```python
from build123d import *

# Parameters (mm, degrees)
BOSS_EXTRUDE1_DEPTH             = 2
BOSS_EXTRUDE3_DEPTH             = 8
BOSS_EXTRUDE2_REACH             = 28
BOSS_EXTRUDE2_DIRECTION_2_REACH = 28
TAP_DRILL_FOR_M3X0_5_TAP1_D     = 2.5
TAP_DRILL_FOR_M3X0_5_TAP1_DEPTH = 8


with BuildPart() as part:
    # Sketch1 → Boss-Extrude1 (new body)
    with BuildSketch(Plane(origin=(0, 0, 0), x_dir=(1, 0, 0), z_dir=(0, 1, 0))):
        with BuildLine():
            Line((-26, 0), (-26, -19))
            Line((-26, -19), (26, -19))
            Line((26, -19), (26, 0))
            ThreePointArc((26, 0), (0, 26), (-26, 0))
        make_face()
    extrude(amount=BOSS_EXTRUDE1_DEPTH)

    # Sketch1<3> → Boss-Extrude3 (add)
    with BuildSketch(Plane(origin=(0, 0, 0), x_dir=(1, 0, 0), z_dir=(0, 1, 0))):
        with BuildLine():
            ThreePointArc((26, 0), (0, 26), (-26, 0))
            Line((-26, 0), (-26, -19))
            Line((-26, -19), (26, -19))
            Line((26, -19), (26, 0))
        make_face()
    extrude(amount=BOSS_EXTRUDE3_DEPTH)

    # Boss-Extrude2: up to this face of the body (flat: up to its plane)
    boss_extrude2_end = Plane(part.part.faces().sort_by_distance((26, 4, 9.5))[0])
    # Sketch3 → Boss-Extrude2 (add, up to the picked face)
    with BuildSketch(Plane(origin=(0, 0, 0), x_dir=(0, 0, -1), z_dir=(1, 0, 0)), mode=Mode.PRIVATE) as boss_extrude2_sk1:
        Polygon((-19, 8), (-19, 16.5), (-11, 16.5), (-11, 13.5), (-16, 13.5), (-16, 8), align=None)
    boss_extrude2_tool1 = split(extrude(boss_extrude2_sk1.sketch, amount=BOSS_EXTRUDE2_REACH, mode=Mode.PRIVATE), bisect_by=boss_extrude2_end, keep=Keep.BOTH, mode=Mode.PRIVATE)
    add(boss_extrude2_tool1.solids().sort_by_distance((0, 13.268519, 16.018519))[0])

    # Boss-Extrude2 direction 2: up to this face of the body (flat: up to its plane)
    boss_extrude2_direction_2_end = Plane(part.part.faces().sort_by_distance((-26, 4, 9.5))[0])
    # Sketch3 → Boss-Extrude2 direction 2 (add, up to the picked face)
    with BuildSketch(Plane(origin=(0, 0, 0), x_dir=(0, 0, -1), z_dir=(1, 0, 0)), mode=Mode.PRIVATE) as boss_extrude2_direction_2_sk1:
        Polygon((-19, 8), (-19, 16.5), (-11, 16.5), (-11, 13.5), (-16, 13.5), (-16, 8), align=None)
    boss_extrude2_direction_2_tool1 = split(extrude(boss_extrude2_direction_2_sk1.sketch, amount=-BOSS_EXTRUDE2_DIRECTION_2_REACH, mode=Mode.PRIVATE), bisect_by=boss_extrude2_direction_2_end, keep=Keep.BOTH, mode=Mode.PRIVATE)
    add(boss_extrude2_direction_2_tool1.solids().sort_by_distance((0, 13.268519, 16.018519))[0])

    # Tap Drill for M3x0.5 Tap1
    with Locations(Plane(origin=(0, 0, 0), x_dir=(-1, 0, 0), z_dir=(0, -1, 0))):
        with Locations((-6.75, 11), (6.75, 11), (6.75, -11), (-6.75, -11)):
            Hole(TAP_DRILL_FOR_M3X0_5_TAP1_D / 2, depth=TAP_DRILL_FOR_M3X0_5_TAP1_DEPTH)


solid = part.part
```
Verification items for the finished model (mm, model axes). A direction names the side the tool comes from. Coordinates: 2 decimals unless noted, no trailing zeros. Loops run counter-clockwise (first coordinate to the right, second up) from the corner with the lowest first, then second, coordinate; pieces in that order, holes last. Notation, with made-up numbers: (53.5, 43.5) - (72.5, 43.5) arc R28 ccw to (72.5, 62.5) - close; hole circle Ø2 at (79, 16.5). An arc over 180 degrees is marked (long way). Put each result on its own line as item: value.
Item 1: Section check A-A (x = 0). Enter the section's corners in (y, z), then the cut area to 4 significant figures.
Conclusion:
outline: (0, -26) - (8, -26) - (8, 16) - (13.5, 16) - (13.5, 11) - (16.5, 11) - (16.5, 19) - (0, 19) - close
area: 400.5 mm2
Item 2: Draft check along Z on faces 5 (the face through (0, 8, -1)), 6 (the face through (0, 11, 16)), 7 (the face through (6, 4, -12)). Enter one of: pulls with the +Z half, pulls with the -Z half, needs draft (parallel to the pull), parting line crosses it, or undercut.
Conclusion:
face 5: needs draft
face 6: pulls with the -Z half
face 7: undercut
Item 3: Gauge pin test, flat ends, axial feed: pin 1 Ø4 at (x, z) = (-3.5, 13.5) entering from -Y; pin 2 Ø6 at (x, y) = (12, 11.5) entering from -Z; pin 3 Ø2 at (x, y) = (19.5, 9.5) entering from -Z; pin 4 Ø21 at (x, z) = (10.5, -3) entering from +Y. Record the tip position at first contact, or that the pin passes through.
Conclusion:
pin 1: stops at y = 0
pin 2: stops at z = 11
pin 3: stops at z = 16
pin 4: stops at y = 8
Item 4: Set-up check for faces 1 (the face through (0, 13.5, 13)), 2 (the face through (0, 15, 11)), 3 (the face through (6, 4, 10)), 4 (the face through (-6.91, 4.06, -12.24)): record each of +Z, -Z, +X, -X, +Y, -Y from which the full face is reachable in a straight line by a thin tool's end or side.
Conclusion:
face 1: -Z, +X, -X
face 2: -Z, +X, -X, +Y
face 3: -Y
face 4: +Y, -Y
Item 5: Section check D-D (x = 15.5). Enter the section's corners in (y, z).
Conclusion:
outline: (0, -20.87) - (8, -20.87) - (8, 16) - (13.5, 16) - (13.5, 11) - (16.5, 11) - (16.5, 19) - (0, 19) - close
Item 6: Section check C-C (x = -6.75). Enter the section's corners in (y, z).
Conclusion:
outline: (0, -25.11) - (8, -25.11) - (8, -12.25) - (0, -12.25) - close; (0, -9.75) - (8, -9.75) - (8, 9.75) - (0, 9.75) - close; (0, 12.25) - (8, 12.25) - (8, 16) - (13.5, 16) - (13.5, 11) - (16.5, 11) - (16.5, 19) - (0, 19) - close
Item 7: Section check B-B (z = -11). Enter the section's corners in (x, y), then the cut area to 3 significant figures.
Conclusion:
outline: (-23.56, 0) - (-8, 0) - (-8, 8) - (-23.56, 8) - close; (-5.5, 0) - (5.5, 0) - (5.5, 8) - (-5.5, 8) - close; (8, 0) - (23.56, 0) - (23.56, 8) - (8, 8) - close
area: 337 mm2
Item 8: Scan lines: line 1 along X through (y, z) = (6, 11); line 2 along Z through (x, y) = (-6.75, 4.5); line 3 along X through (y, z) = (6.25, -11). Record each from-to range of solid material in increasing order.
Conclusion:
line 1: x = -26 to -8, -5.5 to 5.5, 8 to 26
line 2: z = -25.11 to -12.25, -9.75 to 9.75, 12.25 to 19
line 3: x = -23.56 to -8, -5.5 to 5.5, 8 to 23.56
